Print and shaded views of the part. All mm, measured from the part's lowest x, y and z. A direction names the side the tool comes from. Give positions to 0.01 mm unless a question says otherwise; leave off trailing zeros. Write each loop counter-clockwise with the first axis right and the second up, starting at its lowest first coordinate (ties: lowest second). Pieces come first, ordered by that corner, then holes. Notation, with made-up numbers: (5, 39.5) -> (37, 39.5) arc R30 cw to (37, 70.5) -> close; hole circle Ø9 at (66, 74.5). An arc over 180 degrees is marked (long way). Put each result on its own line as item: value.
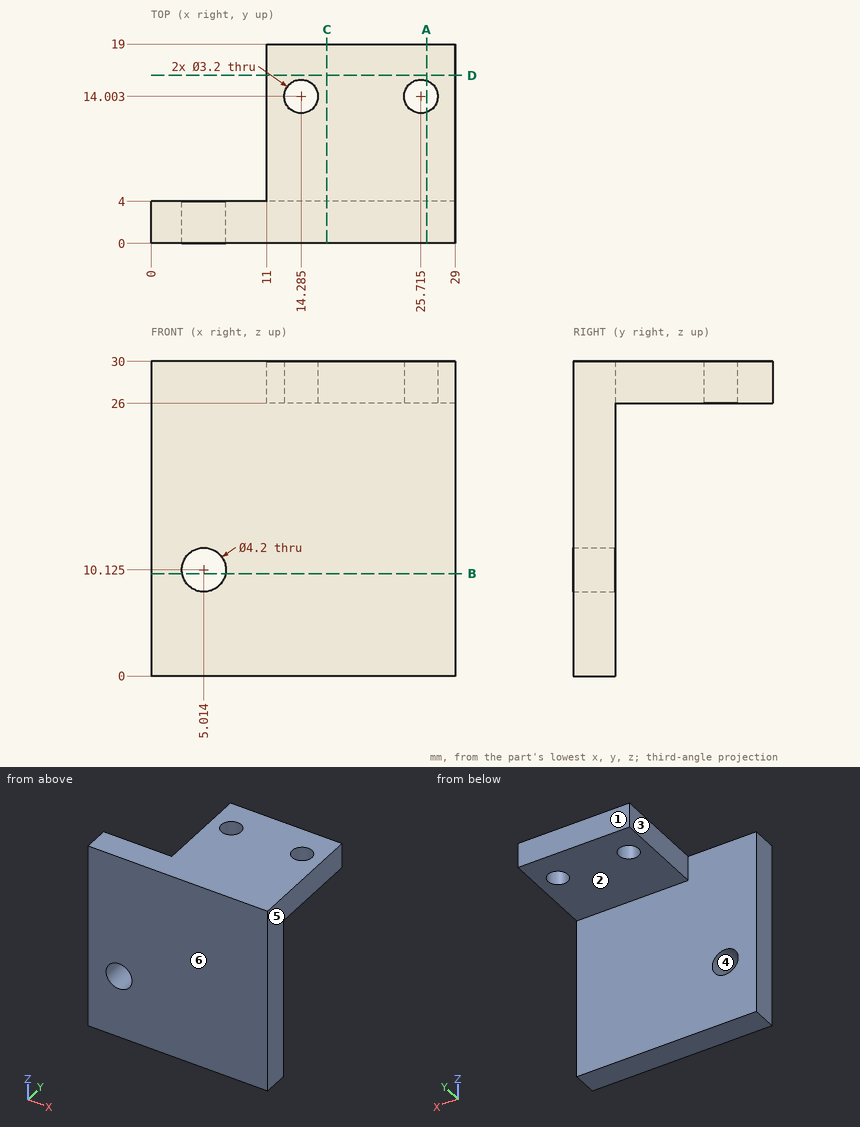
1) Slice it at B-B (z = 9.75). Write the cut outline in (x, y).
Filled sheet:
outline: (0, 0) -> (2.95, 0) -> (2.95, 4) -> (0, 4) -> close; (7.08, 0) -> (29, 0) -> (29, 4) -> (7.08, 4) -> close
2) Slice it at C-C (x = 16.75). Write the cut outline in (y, z), plus the area to 3 significant figures.
Filled sheet:
outline: (0, 0) -> (4, 0) -> (4, 26) -> (19, 26) -> (19, 30) -> (0, 30) -> close
area: 180 mm2
3) Wall check: L1, parallel to Y at x = 2.25, z = 3.25; L2, parallel to Z at x = 11.5, y = 18.25. Give the ranges that are in metal, low to high.
Filled sheet:
L1: 0 to 4
L2: 26 to 30
4) Tool access for the marked faces 1 and 2: list every direction of +Z, -Z, +X, -X, +Y, -Y with a clear straight run to the whole face (end or side of a thin tool).
Filled sheet:
face 1: +Z, -Z, +X, -X, +Y
face 2: -Z, +X, -X, +Y
5) Pull direction X, two halves, no side cores. Call the marked faces 3, 4, 5 and 6: released by +X, released by -X, zero draft, split by the parting line, or undercut.
Filled sheet:
face 3: released by -X
face 4: undercut
face 5: released by +X
face 6: zero draft
6) Pin check, flat tips, straight feed: pin 1 (6 mm diameter, centred on x = 18, z = 20.5, fed in from +Y); pin 2 (4.5 mm diameter, centred on x = 16.5, y = 14.5, fed in from -Z); pin 3 (2 mm diameter, centred on y = 15, z = 27, fed in from -X). Stop position of each tip, or through.
Filled sheet:
pin 1: y = 4
pin 2: z = 26
pin 3: x = 11
7) Slice it at D-D (y = 16). Write the cut outline in (x, z).
Filled sheet:
outline: (11, 26) -> (29, 26) -> (29, 30) -> (11, 30) -> close
8) Slice it at A-A (x = 26.25). Write the cut outline in (y, z) (1 decimal).
Filled sheet:
outline: (0, 0) -> (4, 0) -> (4, 26) -> (12.5, 26) -> (12.5, 30) -> (0, 30) -> close; (15.5, 26) -> (19, 26) -> (19, 30) -> (15.5, 30) -> close
